```python
from build123d import *

# Parameters (mm, degrees)
F0_W     = 9.5
F0_H     = 21.5
F1_DEPTH = 3.5
F2_R     = 1.55
F3_DEPTH = 3.5
F4_W     = 9.5
F4_H     = 8.2
F5_DEPTH = 0.6
F7_DEPTH = 2.3


with BuildPart() as f1:
    # F0 (on Top) → F1 (new body)
    with BuildSketch(Plane.XY):
        Rectangle(F0_W, F0_H)
    extrude(amount=F1_DEPTH)

    # F2 (on face) → F3 (cut, through all)
    with BuildSketch(Plane.XY.offset(3.5)):
        with Locations((0, 7)):
            Circle(F2_R)
        with Locations((0, -7)):
            Circle(F2_R)
    extrude(amount=-F3_DEPTH, mode=Mode.SUBTRACT)

    # F4 (on face) → F5 (cut)
    with BuildSketch(Plane(origin=(0, 0, 0), x_dir=(1, 0, 0), z_dir=(0, 0, -1))):
        Rectangle(F4_W, F4_H)
    extrude(amount=-F5_DEPTH, mode=Mode.SUBTRACT)

    # F6 (on face) → F7 (cut)
    with BuildSketch(Plane.XY.offset(3.5)):
        Polygon((1.587713, 4.25), (3.175426, 7), (1.587713, 9.75), (-1.587713, 9.75), (-3.175426, 7), (-1.587713, 4.25), align=None)
        Polygon((1.587713, -9.75), (3.175426, -7), (1.587713, -4.25), (-1.587713, -4.25), (-3.175426, -7), (-1.587713, -9.75), align=None)
    extrude(amount=-F7_DEPTH, mode=Mode.SUBTRACT)


solid = f1.part
```
For this review, take the finished solid that the model builds, in its own axes (mm). A direction names the side the tool comes from. Give positions to 0.01 mm unless a question says otherwise; leave off trailing zeros. Order: outer loops, then holes, each group sorted by start corner. A loop starts at its lowest first (then second) coordinate and runs counter-clockwise, first axis right, second up.
1) Take a section at C-C (x = -4). Give the boundary of the cut face in (y, z), then the cut area to 3 significant figures.
2) Take a section at B-B (z = 1.95). Give the boundary of the cut face in (x, y).
3) For faces 5 (the face through (-0.336, -8.513, 0.608)), 6 (the face through (-2.37, 8.394, 2.366)), list the 3-axis set-ups (+Z, -Z, +X, -X, +Y, -Y) from which the entire face can be reached by the end or side of a thin tool; tool diameter is ignored.
4) Take a section at D-D (y = -5.25). Give the boundary of the cut face in (x, z), then the cut area to 3 significant figures.
5) Take a section at A-A (x = 0). Give the boundary of the cut face in (y, z).
6) Wall thickness on line 1 (Y direction, x = 0, z = 0.9); line 2 (Y direction, x = -0.25, z = 3.1); line 3 (Y direction, x = 0, z = 0.55): over which ranges is each line inside the solid? List them lowest first.
7) The part is to be moulded in two halves that separate along Y. For faces 1 (the face through (-2.39, -8.36, 2.37)), 2 (the face through (0, 10.75, 2)), 3 (the face through (2.37, -8.394, 2.366)), 4 (the face through (4.75, 0, 2)), say which applies: released by +Y, released by -Y, zero draft, split by the parting line, or undercut.
8) Insertion check: pin 1 (4 mm diameter, centred on x = -2, y = -1.5, fed in from -Z); pin 2 (1.9 mm diameter, centred on x = 0, y = 7, fed in from +Z); pin 3 (4.5 mm diameter, centred on x = 0, y = 7, fed in from +Z). Each pin has a flat end and moves straight along its axis. Give the tip position at first contact, or say it passes through.
Derived:
1. outline: (-10.75, 0) - (-4.1, 0) - (-4.1, 0.6) - (4.1, 0.6) - (4.1, 0) - (10.75, 0) - (10.75, 3.5) - (-10.75, 3.5) - close
1. area: 70.3 mm2
2. outline: (-4.75, -10.75) - (4.75, -10.75) - (4.75, 10.75) - (-4.75, 10.75) - close; hole (-3.18, -7) - (-1.59, -9.75) - (1.59, -9.75) - (3.18, -7) - (1.59, -4.25) - (-1.59, -4.25) - close; hole (-3.18, 7) - (-1.59, 4.25) - (1.59, 4.25) - (3.18, 7) - (1.59, 9.75) - (-1.59, 9.75) - close
3. face 5: +Z, -Z
3. face 6: +Z
4. outline: (-4.75, 0) - (4.75, 0) - (4.75, 3.5) - (2.17, 3.5) - (2.17, 1.2) - (-2.17, 1.2) - (-2.17, 3.5) - (-4.75, 3.5) - close
4. area: 23.3 mm2
5. outline: (-10.75, 0) - (-8.55, 0) - (-8.55, 1.2) - (-9.75, 1.2) - (-9.75, 3.5) - (-10.75, 3.5) - close; (-5.45, 0) - (-4.1, 0) - (-4.1, 0.6) - (4.1, 0.6) - (4.1, 0) - (5.45, 0) - (5.45, 1.2) - (4.25, 1.2) - (4.25, 3.5) - (-4.25, 3.5) - (-4.25, 1.2) - (-5.45, 1.2) - close; (8.55, 0) - (10.75, 0) - (10.75, 3.5) - (9.75, 3.5) - (9.75, 1.2) - (8.55, 1.2) - close
6. line 1: y = -10.75 to -8.55, -5.45 to 5.45, 8.55 to 10.75
6. line 2: y = -10.75 to -9.75, -4.25 to 4.25, 9.75 to 10.75
6. line 3: y = -10.75 to -8.55, -5.45 to -4.1, 4.1 to 5.45, 8.55 to 10.75
7. face 1: undercut
7. face 2: released by +Y
7. face 3: undercut
7. face 4: zero draft
8. pin 1: stops at z = 0.6
8. pin 2: passes through
8. pin 3: stops at z = 1.2
